from build123d import *

# Parameters (mm, degrees)
F0_W     = 46.632492
F0_H     = 83.48006
F0_W_2   = 41.954536
F0_H_2   = 78.36432
F1_DEPTH = 25.4
F2_W     = 25.159884
F2_H     = 7.646168
F3_DEPTH = 76.2
F5_DEPTH = 127


with BuildPart() as f1:
    # F0 (on Top) → F1 (new body)
    with BuildSketch(Plane.XY):
        Rectangle(F0_W, F0_H)
        Rectangle(F0_W_2, F0_H_2, mode=Mode.SUBTRACT)
    extrude(amount=F1_DEPTH)

    # F2 (on face) → F3 (cut)
    with BuildSketch(Plane.YZ.offset(23.316246)):
        with Locations((0, 21.576916)):
            Rectangle(F2_W, F2_H)
    extrude(amount=-F3_DEPTH, mode=Mode.SUBTRACT)

    # F4 (on face) → F5 (cut)
    with BuildSketch(Plane.XZ.offset(41.74003)):
        with BuildLine():
            Line((0, 17.130356), (0, 8.269644))
            ThreePointArc((0, 8.269644), (3.132735, 9.567265), (4.430356, 12.7))
            ThreePointArc((4.430356, 12.7), (3.132735, 15.832735), (0, 17.130356))
        make_face()
        with BuildLine():
            ThreePointArc((0, 17.130356), (-4.430356, 12.7), (0, 8.269644))
            Line((0, 8.269644), (0, 17.130356))
        make_face()
    extrude(amount=-F5_DEPTH, mode=Mode.SUBTRACT)


solid = f1.part
Read the model definition and answer for the solid it produces. Units are mm, in the model's axes. A direction names the side the tool comes from. Give positions to 0.01 mm unless a question says otherwise; leave off trailing zeros. Write each loop counter-clockwise with the first axis right and the second up, starting at its lowest first coordinate (ties: lowest second). Pieces come first, ordered by that corner, then holes. Notation, with made-up numbers: (3, 22.5) - (22, 22.5) arc R19 cw to (22, 49.5) - close; hole circle Ø11 at (41, 88). An arc over 180 degrees is marked (long way). Use CSV: the item, a comma, the result in double quotes. Start each with the question number.
(1) Determine the mould class of faces 1 (the flat face through (22, 0, 17.754)), 2 (the flat face through (-20.977, -1, 13)), 3 (the flat face through (-23.316, -1, 13)) for opening direction X: +X half, -X half, draft (parallel to the pull), parting line (faces both ways), or undercut.
(2) Find section C-C (x = 18.5). Give the vertices of the cut face in (y, z), plus the area to 3 significant figures.
(3) For faces 4 (the flat face through (-5, 39.182, 13)), 5 (the flat face through (0, -40, 25.4)), 6 (the flat face through (22, -12.58, 22)), determine the directions among +Z, -Z, +X, -X, +Y, -Y from which every point of the face is accessible in a straight line to the end or side of a thin tool.
(4) Given P1, Ø1.9, axis at x = -22.5, y = 1, coming from the +Z side; P2, Ø12, axis at x = 11.5, y = 17.5, coming from the +Z side, each flat-ended and moving along its own axis, determine where each tip first touches the part or whether it passes through.
(5) Find section A-A (y = -8). Give the vertices of the cut face in (x, z), plus the area to 3 significant figures.
(6) Find section D-D (z = 6.25). Give the vertices of the cut face in (x, y).
(7) Find section B-B (z = 23.75). Give the vertices of the cut face in (x, y).
(8) Consider line 1 along Y through (x, z) = (5.5, 6); line 2 along X through (y, z) = (26.5, 6). Determine where each line is inside the solid, lowest interval first.
Findings below:
1,face 1,"draft"
1,face 2,"undercut"
1,face 3,"-X half"
2,outline,"(-41.74, 0) - (-39.18, 0) - (-39.18, 25.4) - (-41.74, 25.4) - close; (39.18, 0) - (41.74, 0) - (41.74, 25.4) - (39.18, 25.4) - close"
2,area,"130 mm2"
3,face 4,"+Z, -Z"
3,face 5,"+Z, +X, -X, +Y, -Y"
3,face 6,"+Z, +X, -X"
4,P1,"z = 17.75"
4,P2,"through"
5,outline,"(-23.32, 0) - (-20.98, 0) - (-20.98, 17.75) - (-23.32, 17.75) - close; (20.98, 0) - (23.32, 0) - (23.32, 17.75) - (20.98, 17.75) - close"
5,area,"83.1 mm2"
6,outline,"(-23.32, -41.74) - (23.32, -41.74) - (23.32, 41.74) - (-23.32, 41.74) - close; hole (-20.98, -39.18) - (20.98, -39.18) - (20.98, 39.18) - (-20.98, 39.18) - close"
7,outline,"(-23.32, -41.74) - (23.32, -41.74) - (23.32, -12.58) - (20.98, -12.58) - (20.98, -39.18) - (-20.98, -39.18) - (-20.98, -12.58) - (-23.32, -12.58) - close; (-23.32, 12.58) - (-20.98, 12.58) - (-20.98, 39.18) - (20.98, 39.18) - (20.98, 12.58) - (23.32, 12.58) - (23.32, 41.74) - (-23.32, 41.74) - close"
8,line 1,"-41.74 to -39.18, 39.18 to 41.74"
8,line 2,"-23.32 to -20.98, 20.98 to 23.32"
